The model under review builds one solid part; all positions refer to its coordinate system, in mm. A direction names the side the tool comes from. Give positions to 0.01 mm unless a question says otherwise; leave off trailing zeros. Order: outer loops, then holes, each group sorted by start corner. A loop starts at its lowest first (then second) coordinate and runs counter-clockwise, first axis right, second up. Notation, with made-up numbers: (-5, 38.25) - (22, 38.25) arc R26 cw to (22, 70.25) - close; hole circle Ø9 at (15, 15). An arc over 180 degrees is marked (long way). Put each result on its own line as item: value.
```python
from build123d import *

# Parameters (mm, degrees)
SKETCH1_R           = 6.35
BOSS_EXTRUDE1_DEPTH = 33.7312
SKETCH2_W           = 20.748446766
SKETCH2_H           = 0.9906
SKETCH3_W           = 15.336822943
SKETCH3_H           = 0.9906
CUT_EXTRUDE1_DEPTH  = 1.778


with BuildPart() as part:
    # Sketch1 → Boss-Extrude1 (new body)
    with BuildSketch(Plane(origin=(0, 0, 0), x_dir=(1, 0, 0), z_dir=(0, 1, 0))):
        Circle(SKETCH1_R)
    extrude(amount=BOSS_EXTRUDE1_DEPTH)

    # Sketch2 → Cut-Revolve1 (revolve, cut)
    with BuildSketch(Plane(origin=(0, 0, 0), x_dir=(0, 0, -1), z_dir=(1, 0, 0))):
        with Locations((-16.317823383, 23.7109)):
            Rectangle(SKETCH2_W, SKETCH2_H)
    revolve(axis=Axis((0, 25.517050234, 0), (0, -1, 0)), mode=Mode.SUBTRACT)

    # Sketch3 → Cut-Revolve2 (revolve, cut)
    with BuildSketch(Plane(origin=(0, 0, 0), x_dir=(0, 0, -1), z_dir=(1, 0, 0))):
        with Locations((-13.612011472, 10.0203)):
            Rectangle(SKETCH3_W, SKETCH3_H)
    revolve(axis=Axis((0, 15.810643297, 0), (0, -1, 0)), mode=Mode.SUBTRACT)

    # Sketch4 → Cut-Extrude1 (cut)
    with BuildSketch(Plane(origin=(6.35, 0, 0), x_dir=(0, 0, -1), z_dir=(1, 0, 0))):
        with BuildLine():
            Line((1.5875, 23.2156), (1.5875, 10.5156))
            ThreePointArc((1.5875, 10.5156), (0, 8.9281), (-1.5875, 10.5156))
            Line((-1.5875, 10.5156), (-1.5875, 23.2156))
            ThreePointArc((-1.5875, 23.2156), (0, 24.8031), (1.5875, 23.2156))
        make_face()
    extrude(amount=-CUT_EXTRUDE1_DEPTH, mode=Mode.SUBTRACT)


solid = part.part
```
(1) The part is to be moulded in two halves that separate along Z. For faces 1 (the cylindrical face through (5.28, 8.93, -0.03)), 2 (the cylindrical face through (-1.38, 28.9, 6.2)), 3 (the flat face through (4.572, 17, 0)), 4 (the flat face through (-6.1, 9.525, 0)), say which applies: pulls with the +Z half, pulls with the -Z half, needs draft (parallel to the pull), parting line crosses it, or undercut.
The answers:
face 1: undercut
face 2: parting line crosses it
face 3: undercut
face 4: needs draft
(2) Take a section at A-A, the plane z = 0. Write out the cut boundary in (x, y) (3 decimals).
The answers:
outline: (-6.35, 0) - (6.35, 0) - (6.35, 8.928) - (4.572, 8.928) - (4.572, 24.803) - (6.35, 24.803) - (6.35, 33.731) - (-6.35, 33.731) - (-6.35, 24.206) - (-5.944, 24.206) - (-5.944, 23.216) - (-6.35, 23.216) - (-6.35, 10.516) - (-5.944, 10.516) - (-5.944, 9.525) - (-6.35, 9.525) - close
(3) Wall thickness on L1, parallel to Y at x = -5.75, z = 2.25 (3 decimals); L2, parallel to X at y = 22.5, z = 0.25; L3, parallel to Z at x = 2.25, y = 4: over which ranges is each line inside the solid? List them lowest first.
The answers:
L1: 0 to 9.525, 10.516 to 23.216, 24.206 to 33.731
L2: -6.35 to 4.57
L3: -5.94 to 5.94
(4) Take a section at D-D, the plane z = 4. Write out the cut boundary in (x, y) (3 decimals).
The answers:
outline: (-4.932, 0) - (4.932, 0) - (4.932, 9.525) - (4.396, 9.525) - (4.396, 10.516) - (4.932, 10.516) - (4.932, 23.216) - (4.396, 23.216) - (4.396, 24.206) - (4.932, 24.206) - (4.932, 33.731) - (-4.932, 33.731) - (-4.932, 24.206) - (-4.396, 24.206) - (-4.396, 23.216) - (-4.932, 23.216) - (-4.932, 10.516) - (-4.396, 10.516) - (-4.396, 9.525) - (-4.932, 9.525) - close
(5) For faces 5 (the flat face through (0, 33.731, 0)), 6 (the flat face through (5, 17, -1.588)), 7 (the flat face through (-6.1, 24.206, 0)), list the 3-axis set-ups (+Z, -Z, +X, -X, +Y, -Y) from which the entire face can be reached by the end or side of a thin tool; tool diameter is ignored.
The answers:
face 5: +Z, -Z, +X, -X, +Y
face 6: +X
face 7: none
(6) Clearance check with flat-ended pins moving along their axes: pin 1 Ø1 at (y, z) = (6.5, -3) entering from +X; pin 2 Ø1.6 at (y, z) = (16, 0.5) entering from +X; pin 3 Ø1.5 at (x, y) = (5, 21.5) entering from +Z. State where each tip first meets the part, or that it passes through.
The answers:
pin 1: x = 5.84
pin 2: x = 4.57
pin 3: z = 4.72
(7) Take a section at B-B, the plane x = 3.5. Write out the cut boundary in (y, z) (3 decimals).
The answers:
outline: (0, -5.298) - (9.525, -5.298) - (9.525, -4.804) - (10.516, -4.804) - (10.516, -5.298) - (23.216, -5.298) - (23.216, -4.804) - (24.206, -4.804) - (24.206, -5.298) - (33.731, -5.298) - (33.731, 5.298) - (24.206, 5.298) - (24.206, 4.804) - (23.216, 4.804) - (23.216, 5.298) - (10.516, 5.298) - (10.516, 4.804) - (9.525, 4.804) - (9.525, 5.298) - (0, 5.298) - close
(8) Take a section at C-C, the plane y = 6.5. Write out the cut boundary in (x, z), then the cut area to 3 significant figures.
The answers:
outline: circle Ø12.7 at (0, 0)
area: 127 mm^2
